Source: CAD feature listing. Evaluate the final solid. Frame: model axes, mm. A direction names the side the tool comes from. Coordinates: 2 decimals unless noted, no trailing zeros. Order: outer loops, then holes, each group sorted by start corner. A loop starts at its lowest first (then second) coordinate and runs counter-clockwise, first axis right, second up. Notation, with made-up numbers: (21, 62.5) -> (25, 62.5) arc R15 cw to (25, 72.5) -> close; hole circle Ø3 at (4, 81.25). An arc over 180 degrees is marked (long way). Put each result on its own line as item: value.
Autodesk Inventor part; units mm, degrees
ref_plane "YZ Plane" through (0, 0, 0) normal (1, 0, 0) x (0, 1, 0)
ref_plane "XZ Plane" through (0, 0, 0) normal (0, 1, 0) x (-1, 0, 0)
ref_plane "XY Plane" through (0, 0, 0) normal (0, 0, 1) x (1, 0, 0)
sketch "Sketch1" plane through (0, 0, 0) normal (0, 0, 1) x (1, 0, 0)
  line L0 (0, 0) -> (0, 137.0131)
  line L1 (-11.7886, 12.2907) -> (-39.6863, 18.4755) construction
  line L2 (-39.6863, 18.4755) -> (-33.3297, 47.1481) construction
  line L3 (-33.3297, 47.1481) -> (-5.432, 40.9633) construction
  line L4 (-5.432, 40.9633) -> (-11.7886, 12.2907) construction
  line L5 (-39.6863, 18.4755) -> (-5.432, 40.9633) construction
  line L6 (-33.3297, 47.1481) -> (-11.7886, 12.2907) construction
  circle A0 centre (-53.975, 12.7) radius 3.175
  circle A1 centre (-53.975, 12.7) radius 9.525
  line L7 (0, 0) -> (-54.5315, 3.1913) construction
  line L8 (-62.4238, 17.0982) -> (0, 137.0131)
  line L9 (-27.1302, 45.7737) -> (-37.4529, 28.5497) construction
  line L10 (-11.6315, 42.3377) -> (-9.5552, 22.3649) construction
  line L11 (-19.3809, 44.0557) -> (-25.7374, 15.3831) construction
  line L12 (0, 104.775) -> (-15.0457, 108.1106)
  line L13 (-35.3766, 8.5768) -> (-19.8779, 5.1408) construction
  line L14 (-19.8779, 5.1408) -> (-21.2523, -1.0586) construction
  line L15 (-21.2523, -1.0586) -> (-36.751, 2.3773) construction
  line L16 (-36.751, 2.3773) -> (-35.3766, 8.5768) construction
  line L17 (-35.3766, 8.5768) -> (-44.7305, 2.6177) construction
  line L18 (-19.8779, 5.1408) -> (-17.2457, 1.0092) construction
  line L19 (-5.432, 40.9633) -> (-33.3297, 47.1481) construction
  line L20 (-33.3297, 47.1481) -> (-32.2475, 52.0296) construction
  line L21 (-32.2475, 52.0296) -> (-4.3498, 45.8448) construction
  line L22 (-4.3498, 45.8448) -> (-5.432, 40.9633) construction
  line L23 (-53.2878, 15.7997) -> (-53.975, 12.7) construction
  line L24 (-53.975, 12.7) -> (-57.0747, 13.3872) construction
  line L25 (-27.6272, 6.8588) -> (-34.4992, -24.1386) construction
  line L26 (-31.8676, 50.076) -> (-5.5198, 44.2349) construction
  line L27 (-5.5198, 44.2349) -> (-4.489, 48.8845) construction
  line L28 (-4.489, 48.8845) -> (-30.8368, 54.7256) construction
  line L29 (-30.8368, 54.7256) -> (-31.8676, 50.076) construction
  line L30 (-31.3522, 52.4008) -> (-5.0044, 46.5597) construction
  circle A2 centre (-29.0274, 51.8854) radius 1.4732 construction
  circle A3 centre (-22.8279, 50.5111) radius 1.4732 construction
  circle A4 centre (-16.6284, 49.1367) radius 1.4732
  circle A5 centre (-10.4289, 47.7623) radius 1.4732
  circle A6 centre (-7.6985, 96.7513) radius 1.4732
  line L31 (-53.975, 12.7) -> (-5.4185, 105.9762)
  line L32 (-31.2085, 56.4341) -> (0, 49.5153)
  circle A7 centre (-7.6985, 96.7513) radius 4.7625
  line L33 (-4.7625, 50.5712) -> (-4.7625, 105.8308)
  line L34 (-26.3948, 55.3669) -> (-7.323, 92.0036)
  line L35 (-3.5958, 94.3328) -> (-4.7625, 94.5914) construction
  line L36 (-17.2457, 1.0092) -> (0, 1.0092) construction
  line L37 (0, 1.0092) -> (0, -2.1658) construction
  line L38 (0, -2.1658) -> (-17.2457, -2.1658) construction
  line L39 (-17.2457, -2.1658) -> (-17.2457, 1.0092) construction
  circle A8 centre (-12.7, 7.9375) radius 1.5875 construction
  line L40 (-12.7, 7.9375) -> (0, 7.9375) construction
  line L41 (0, 7.9375) -> (-17.2457, 1.0092)
  circle A9 centre (-12.7, 7.9375) radius 3.175 construction
  line L42 (-9.525, 7.9375) -> (-9.525, 4.111) construction
  line L43 (-9.525, 7.9375) -> (0, 7.9375) construction
  line L44 (-17.9187, 46.9837) -> (-16.8879, 51.6333) construction
  line L45 (-12.4942, 45.7811) -> (-26.2381, -16.2137) construction
  line L46 (0, 53.6985) -> (0, 7.9375) construction
  line L47 (-26.2381, -16.2137) -> (-20.0386, -17.5881) construction
  line L48 (-20.0386, -17.5881) -> (-8.7313, 7.9375)
  circle A10 centre (-12.7, 6.35) radius 1.4224
  line L49 (0, 13.4938) -> (-4.7625, 13.4938) construction
  line L50 (-4.7625, 13.4938) -> (-4.7625, 24.6063) construction
  line L51 (-4.7625, 24.6063) -> (0, 24.6063) construction
  line L52 (0, 24.6063) -> (0, 13.4938) construction
  line L53 (-4.7625, 19.05) -> (0, 19.05) construction
  circle A11 centre (-2.3813, 19.05) radius 1.4224
  line L54 (-20.7405, 8.5842) -> (-9.7454, 58.18) construction
  line L55 (-9.7454, 58.18) -> (-3.5459, 56.8056) construction
  line L56 (-3.5459, 56.8056) -> (-14.5411, 7.2098) construction
  line L57 (-14.5411, 7.2098) -> (-20.7405, 8.5842) construction
  line L58 (-12.7, 6.35) -> (-12.7, 7.9375) construction
  line L59 (-11.5442, 1.5875) -> (-9.525, 1.5875) construction
  line L60 (-9.525, 1.5875) -> (-9.525, 7.9375) construction
  line L61 (-9.525, 7.9375) -> (-11.5442, 7.9375) construction
  line L62 (-11.5442, 7.9375) -> (-11.5442, 1.5875) construction
  line L63 (-9.7454, 58.18) -> (-15.9449, 59.5544) construction
  line L64 (-18.8691, 53.6985) -> (0, 53.6985)
  line L65 (-9.7454, 58.18) -> (-17.3193, 53.3549) construction
  arc A12 (-10.2313, 55.9882) -> (-11.9373, 58.6659) centre (-11.0843, 57.3271) ccw construction
  line L66 (-4.7625, 57.15) -> (0, 57.15) construction
  circle A13 centre (-2.3813, 57.15) radius 1.4224
  circle A14 centre (-2.3813, 63.5) radius 1.4224
  line L67 (0, 7.9375) -> (-38.5755, 7.9375) construction
  line L68 (-38.5755, 7.9375) -> (-38.5755, -42.8625) construction
  line L69 (-38.5755, -42.8625) -> (0, -42.8625)
  line L70 (0, -42.8625) -> (0, 7.9375)
  line L71 (-38.5755, -42.8625) -> (-62.6076, 8.6746)
  line L72 (-60.0032, 20.0747) -> (-18.8691, 53.6985)
  line L73 (-20.0386, -17.5881) -> (-20.0386, -42.8625) construction
  line L74 (-20.2435, 47.4991) -> (-19.2127, 52.1487) construction
  line L75 (-12.7, -42.8625) -> (-12.7, -1.0217)
  circle A15 centre (-23.8125, -33.3375) radius 1.7526
  circle A16 centre (-15.875, -28.575) radius 1.7526
  circle A17 centre (-23.8125, -33.3375) radius 3.175 construction
  circle A18 centre (-2.3813, 69.85) radius 1.4224
  circle A19 centre (-2.3813, 76.2) radius 1.4224
  circle A20 centre (-15.875, -28.575) radius 3.175 construction
  circle A21 centre (-46.0375, -19.05) radius 1.7526
  arc A22 (0, 104.775) -> (-15.0457, 108.1106) centre (-7.9697, 104.427) ccw
  circle A23 centre (-7.9697, 104.427) radius 1.4224
  line L76 (-7.9697, 104.427) -> (-15.0457, 108.1106) construction
  line L77 (-7.9697, 104.427) -> (0, 104.775) construction
  line L78 (-14.2148, 89.0787) -> (-22.6636, 93.4768)
  point P0 (-22.5591, 29.7194)
  point P1 (-20.7484, 1.2142)
  point P2 (-36.3367, 4.2458)
  point P3 (-49.5768, 21.1488)
  point P4 (-11.1125, 7.9375)
  point P5 (-11.4283, 6.9872)
  point P6 (-11.9574, 7.9375)
  point P7 (-13.9717, 6.9872)
  point P8 (-9.525, 6.1457)
  point P9 (-10.6215, 3.6705)
  point P10 (-4.7625, 93.0015)
  point P11 (-4.7625, 53.6985)
  dimension "d74" = 6.35
  dimension "d14" = 29.3687
  dimension "d15" = 28.575
  dimension "d16" = 12.5
  dimension "d17" = 6.35
  dimension "d19" = 53.975
  dimension "d22" = 19.05
  dimension "d23" = 7.9375
  dimension "d24" = 19.05
  dimension "d26" = 102.5
  dimension "d29" = 6.35
  dimension "d31" = 7.9375
  dimension "d34" = 5
  dimension "d35" = 26.9875
  dimension "d38" = 31.75
  dimension "d40" = 26.9875
  dimension "d41" = 4.7625
  dimension "d42" = 2.9464
  dimension "d43" = 2.3813
  dimension "d46" = 6.35
  dimension "d51" = 2.9464
  dimension "d52" = 92.075
  dimension "d53" = 6.35
  dimension "d54" = 9.525
  dimension "d55" = 4.7625
  dimension "d56" = 4.7625
  dimension "d60" = 12.7
  dimension "d61" = 3.175
  dimension "d63" = 3.175
  dimension "d66" = 3.175
  dimension "d67" = 12.7
  dimension "d72" = 8.7312
  dimension "d73" = 7.9375
  dimension "d80" = 12.7
  dimension "d82" = 7.9375
  dimension "d83" = 63.5
  dimension "d85" = 6.35
  dimension "d86" = 104.775
  dimension "d87" = 2.8448
  dimension "d88" = 4.7625
  dimension "d89" = 11.1125
  dimension "d90" = 2.8448
  dimension "d91" = 19.05
  dimension "d92" = 6.35
  dimension "d93" = 50.8
  dimension "d94" = 25.4
  dimension "d95" = 8.7312
  dimension "d96" = 9.525
  dimension "d97" = 6.35
  dimension "d99" = 6.35
  dimension "d101" = 3.175
  dimension "d106" = 2.8448
  dimension "d107" = 57.15
  dimension "d110" = 6.35
  dimension "d136" = 3.175
  dimension "d138" = 42.8625
  dimension "d139" = 12.7
  dimension "d140" = 3.5052
  dimension "d141" = 3.5052
  dimension "d142" = 9.525
  dimension "d143" = 3.175
  dimension "d144" = 11.1125
  dimension "d145" = 6.35
  dimension "d146" = 14.2875
  dimension "d149" = 6.35
extrude "Extrusion1" add sketch "Sketch1" along normal blind 6.35 contours L70 L69 L75 L48 L41 L0 | L41 L48 L75 L69 L71 A1 L31 L72 L32 L0 | L32 L33 L64 L0 | L64 L33 A7 L12 L0 | L32 L64 L33 | L12 A22 | L72 L31 L32 | A1 | L33 A7 L31 L12 | L12 L31 A7 L78 L8 | L33 A7 | A7 L31 L33 | L32 L31 A7 L34 | L31 A7
fillet "Fillet6" radius 12.7 1 edges at (-38.5755, -42.8625, 3.175)
fillet "Fillet7" radius 6.35 3 edges at (-22.6636, 93.4768, 3.175) (-14.2148, 89.0787, 3.175) (-49.5768, 21.1488, 3.175)
fillet "Fillet8" radius 4.7625 5 edges at (-4.7625, 93.0015, 3.175) (-7.323, 92.0036, 3.175) (-26.3948, 55.3669, 3.175) (-18.8691, 53.6985, 3.175) (-4.7625, 53.6985, 3.175)
equation "\"d56\" = d55"
properties part number "Uprights" material "UHMW, White"
1. Cut plane C-C on z = 4. Count the separate pieces of the cut face and the enclosed holes in it, plus the area to 3 significant figures.
Numbers:
separate pieces: 1
enclosed holes: 15
area: 5,420 mm2
2. Ray query, line 1 along Y through (x, z) = (-12, 0.5); line 2 along Y through (x, z) = (-12.5, 4); line 3 along X through (y, z) = (76, 5). Return the intervals inside material, ascending.
Numbers:
line 1: y = -42.86 to 5.11, 7.59 to 53.7, 81.53 to 111.31
line 2: y = -42.86 to 4.94, 7.76 to 53.7, 81.18 to 110.99
line 3: x = -21.02 to -15.65, -4.76 to -3.79, -0.97 to 0
3. Cut plane B-B on x = -55. Output: boundary loops of the cut face in (y, z) (3 decimals), plus the area to 3 significant figures.
Numbers:
outline: (-7.64, 0) -> (9.695, 0) -> (9.695, 6.35) -> (-7.64, 6.35) -> close; (15.705, 0) -> (22.17, 0) -> (22.17, 6.35) -> (15.705, 6.35) -> close
area: 151 mm2
4. Cut plane D-D on y = 31. Output: boundary loops of the cut face in (x, z), plus the area to 3 significant figures.
Numbers:
outline: (-44.45, 0) -> (0, 0) -> (0, 6.35) -> (-44.45, 6.35) -> close
area: 282 mm2
5. Pull-direction query (X, two-part tool) for faces 3 (the cylindrical face through (-6.386, 112.246, 3.131)), 4 (the cylindrical face through (-57.147, 12.56, 3.131)), 5 (the cylindrical face through (-37.39, -40.82, 3.22)); classes: pulls with the +X half, pulls with the -X half, needs draft (parallel to the pull), parting line crosses it, or undercut.
Numbers:
face 3: parting line crosses it
face 4: undercut
face 5: pulls with the -X half
6. Cut plane A-A on y = 12.7. Output: boundary loops of the cut face in (x, z).
Numbers:
outline: (-63.5, 0) -> (-57.15, 0) -> (-57.15, 6.35) -> (-63.5, 6.35) -> close; (-50.8, 0) -> (0, 0) -> (0, 6.35) -> (-50.8, 6.35) -> close
7. First-contact query: pin 1 (4.5 mm diameter, centred on x = -2.38, y = 63.5, fed in from -Z); pin 2 (4 mm diameter, centred on x = -53.975, y = 12.7, fed in from +Z); pin 3 (3 mm diameter, centred on x = -13.5, z = 3, fed in from +Y). Flat tips, straight axial feed; report the tip coordinate or a pass-through.
Numbers:
pin 1: stops at z = 0
pin 2: passes through
pin 3: stops at y = 111.31
8. Set-up query: faces 1 (the flat face through (-25, 19, 0)), 2 (the cylindrical face through (-6.19, 55.06, 3.22)). Return all of +Z, -Z, +X, -X, +Y, -Y with unobstructed straight access to the full face (end or side cutting, diameter ignored); none if empty.
Numbers:
face 1: -Z, +X, -X, +Y, -Y
face 2: +Z, -Z
